For this review, take the finished solid that the model builds, in its own axes (mm). Coordinates: 2 decimals unless noted, no trailing zeros. Write each loop counter-clockwise with the first axis right and the second up, starting at its lowest first coordinate (ties: lowest second). Pieces come first, ordered by that corner, then holes.
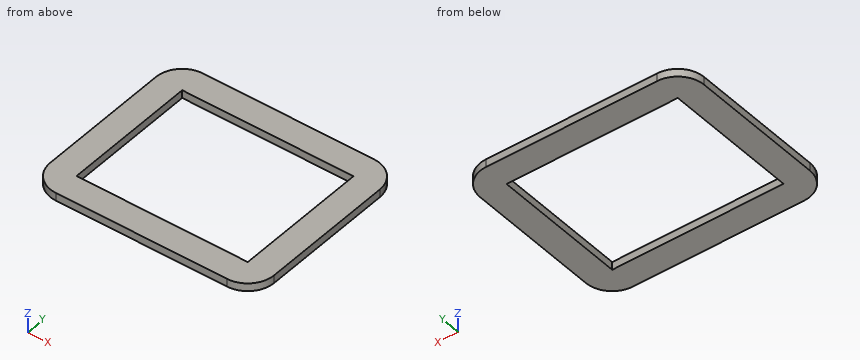
Autodesk Inventor part; units mm, degrees
ref_plane "YZ Plane" through (0, 0, 0) normal (1, 0, 0) x (0, 1, 0)
ref_plane "XZ Plane" through (0, 0, 0) normal (0, 1, 0) x (-1, 0, 0)
ref_plane "XY Plane" through (0, 0, 0) normal (0, 0, 1) x (1, 0, 0)
sketch "Sketch1" plane through (0, 0, 0) normal (0, 0, 1) x (1, 0, 0)
  line L0 (-32.5, 25.5) -> (32.5, 25.5)
  line L1 (32.5, 25.5) -> (32.5, -25.5)
  line L2 (32.5, -25.5) -> (-32.5, -25.5)
  line L3 (-32.5, -25.5) -> (-32.5, 25.5)
  line L4 (-32.5, 35.5) -> (32.5, 35.5)
  line L5 (42.5, 25.5) -> (42.5, -25.5)
  line L6 (32.5, -35.5) -> (-32.5, -35.5)
  line L7 (-42.5, -25.5) -> (-42.5, 25.5)
  arc A0 (-32.5, 35.5) -> (-42.5, 25.5) centre (-32.5, 25.5) ccw
  arc A1 (-42.5, -25.5) -> (-32.5, -35.5) centre (-32.5, -25.5) ccw
  arc A2 (32.5, -35.5) -> (42.5, -25.5) centre (32.5, -25.5) ccw
  arc A3 (42.5, 25.5) -> (32.5, 35.5) centre (32.5, 25.5) ccw
  point P0 (0, 0)
  point P1 (0, 25.5)
  point P2 (32.5, 0)
  point P3 (42.5, 0)
  point P4 (0, 35.5)
  dimension "d0" = 65
  dimension "d1" = 51
  dimension "d2" = 10
  dimension "d3" = 10
  dimension "d4" = 10
extrude "Extrusion1" add sketch "Sketch1" along normal blind 3
equation "\"d4\" = d3"
properties part number "Front_stopper2" material "Polycarbonate, Clear"
Q1. Add section C-C (x = 0.5). State the section outline as (y, z) points, then the cut area to 3 significant figures.
Ans:
outline: (-35.5, 0) - (-25.5, 0) - (-25.5, 3) - (-35.5, 3) - close; (25.5, 0) - (35.5, 0) - (35.5, 3) - (25.5, 3) - close
area: 60.0 mm2
Q2. Add section D-D (x = -36.5). State the section outline as (y, z) points.
Ans:
outline: (-34.67, 0) - (34.67, 0) - (34.67, 3) - (-34.67, 3) - close
Q3. For probe 1 along X at (y, z) = (-5.5, 0.95); probe 2 along Y at (x, z) = (-20.5, 1.45); probe 3 along X at (y, z) = (-26, 2), list the stretches that pass through material, from the lowest coordinate up.
Ans:
probe 1: x = -42.5 to -32.5, 32.5 to 42.5
probe 2: y = -35.5 to -25.5, 25.5 to 35.5
probe 3: x = -42.49 to 42.49
Q4. Add section A-A (y = 14.5). State the section outline as (x, z) points, then the cut area to 3 significant figures.
Ans:
outline: (-42.5, 0) - (-32.5, 0) - (-32.5, 3) - (-42.5, 3) - close; (32.5, 0) - (42.5, 0) - (42.5, 3) - (32.5, 3) - close
area: 60.0 mm2
Q5. Add section B-B (z = 2). State the section outline as (x, y) points.
Ans:
outline: (-42.5, -25.5) arc R10 ccw to (-32.5, -35.5) - (32.5, -35.5) arc R10 ccw to (42.5, -25.5) - (42.5, 25.5) arc R10 ccw to (32.5, 35.5) - (-32.5, 35.5) arc R10 ccw to (-42.5, 25.5) - close; hole (-32.5, -25.5) - (32.5, -25.5) - (32.5, 25.5) - (-32.5, 25.5) - close
